Check sheet for the modelled part. Datum: model origin and axes. Units: mm. A direction names the side the tool comes from. Round coordinates to 2 decimals unless told otherwise and drop trailing zeros. Write each loop counter-clockwise with the first axis right and the second up, starting at its lowest first coordinate (ties: lowest second). Pieces come first, ordered by that corner, then holes.
Item 1: Go/stop test with flat-tipped pins: pin 1 Ø6 at (x, z) = (6.5, -2) entering from -Y; pin 2 Ø0.7 at (x, y) = (1.5, 1) entering from -Z; pin 3 Ø5 at (x, z) = (0, 0.5) entering from -Y; pin 4 Ø2.5 at (x, z) = (0, 0) entering from -Y (3 decimals). Record where each tip stops, or that it passes through.
Item 2: Tool access check on faces 5 (the flat face through (0, 5, -4.95)), 6 (the conical face through (0.025, 0.181, 1.144)). Record the directions out of +Z, -Z, +X, -X, +Y, -Y that give a thin tool (end or side, any length) a straight path to the whole face; none if there is none.
Item 3: Cross-section at A-A on x = 0. Enter the section's corners in (y, z) (3 decimals), plus the area to 3 significant figures.
Item 4: Cross-section at D-D on z = -10.5. Enter the section's corners in (x, y).
Item 5: Material ranges on line 1 (Z direction, x = -0.75, y = 6.5); line 2 (Y direction, x = -2.75, z = -6.25); line 3 (Y direction, x = 5.5, z = -1), recorded low to high.
Item 6: Release check for a two-part mould opening along Z. For faces 1 (the flat face through (-3.39, 5.24, 8.406)), 2 (the flat face through (0, 0, 2)), 3 (the cylindrical face through (0, 1.2, 2.5)), 4 (the flat face through (1.5, 1.2, 0.05)) record: +Z half, -Z half, draft (parallel to the pull), parting line (faces both ways), or undercut.
Item 7: Cross-section at B-B on x = -7.5. Enter the section's corners in (y, z).
Autodesk Inventor part; units mm, degrees
ref_plane "YZ Plane" through (0, 0, 0) normal (1, 0, 0) x (0, 1, 0)
ref_plane "XZ Plane" through (0, 0, 0) normal (0, 1, 0) x (-1, 0, 0)
ref_plane "XY Plane" through (0, 0, 0) normal (0, 0, 1) x (1, 0, 0)
sketch "Sketch1" plane through (0, 0, 0) normal (0, 0, 1) x (1, 0, 0)
  line L0 (0, 7) -> (0, 0) construction
  line L1 (0, 0) -> (1.025, 0) construction
  line L2 (1.025, 0) -> (1.025, 7)
  line L3 (1.025, 7) -> (0, 7) construction
  line L4 (1.025, 7) -> (12, 7)
  line L5 (3, 2.5) -> (2.5, 2.5)
  line L6 (2.5, 2.5) -> (2.5, 0)
  line L7 (2.5, 0) -> (1.025, 0)
  line L8 (12, 7) -> (12, 4.5)
  line L9 (12, 4.5) -> (3, 4.5)
  line L10 (3, 4.5) -> (3, 2.5)
  dimension "d0" = 2.5
  dimension "d1" = 1.025
  dimension "d3" = 0.5
  dimension "d4" = 2.5
  dimension "d9" = 2
  dimension "d10" = 12
  dimension "d11" = 2.5
revolve "Revolution1" add sketch "Sketch1" angle 360 about axis through (0, 7, 0) along (0, -1, 0)
sketch "Sketch2" plane through (0, 7, 0) normal (0, 1, 0) x (1, 0, 0)
  line L0 (0, 0) -> (0, 7.5) construction
  circle A0 centre (0, 7.5) radius 1.35
  line L1 (0, 0) -> (-7.1329, 2.3176) construction
  circle A1 centre (-7.1329, 2.3176) radius 1.35
  line L2 (0, 0) -> (-4.4084, -6.0676) construction
  circle A2 centre (-4.4084, -6.0676) radius 1.35
  line L3 (0, 0) -> (4.4084, -6.0676) construction
  circle A3 centre (4.4084, -6.0676) radius 1.35
  line L4 (0, 0) -> (7.1329, 2.3176) construction
  circle A4 centre (7.1329, 2.3176) radius 1.35
  dimension "d12" = 7.5
  dimension "d13" = 2.7
  dimension "d16" = 360
extrude "Extrusion1" cut sketch "Sketch2" against normal blind 10
sketch "Sketch3" plane through (0, 4.5, 0) normal (0, -1, 0) x (1, 0, 0)
  circle A0 centre (0, -7.5) radius 1.35 construction
  line L0 (-2.9445, -7.5) -> (-1.4722, -4.95)
  line L1 (-1.4722, -4.95) -> (1.4722, -4.95)
  line L2 (1.4722, -4.95) -> (2.9445, -7.5)
  line L3 (2.9445, -7.5) -> (1.4722, -10.05)
  line L4 (1.4722, -10.05) -> (-1.4722, -10.05)
  line L5 (-1.4722, -10.05) -> (-2.9445, -7.5)
  line L6 (6.223, -5.118) -> (4.2528, -2.9298)
  line L7 (4.2528, -2.9298) -> (5.1627, -0.1294)
  line L8 (5.1627, -0.1294) -> (8.0428, 0.4827)
  line L9 (8.0428, 0.4827) -> (10.0131, -1.7054)
  line L10 (10.0131, -1.7054) -> (9.1032, -4.5058)
  line L11 (9.1032, -4.5058) -> (6.223, -5.118)
  line L12 (6.7905, 4.3369) -> (4.1006, 3.1393)
  line L13 (4.1006, 3.1393) -> (1.7185, 4.87)
  line L14 (1.7185, 4.87) -> (2.0262, 7.7984)
  line L15 (2.0262, 7.7984) -> (4.7162, 8.996)
  line L16 (4.7162, 8.996) -> (7.0983, 7.2653)
  line L17 (7.0983, 7.2653) -> (6.7905, 4.3369)
  line L18 (-2.0262, 7.7984) -> (-1.7185, 4.87)
  line L19 (-1.7185, 4.87) -> (-4.1006, 3.1393)
  line L20 (-4.1006, 3.1393) -> (-6.7905, 4.3369)
  line L21 (-6.7905, 4.3369) -> (-7.0983, 7.2653)
  line L22 (-7.0983, 7.2653) -> (-4.7162, 8.996)
  line L23 (-4.7162, 8.996) -> (-2.0262, 7.7984)
  line L24 (-8.0428, 0.4827) -> (-5.1627, -0.1294)
  line L25 (-5.1627, -0.1294) -> (-4.2528, -2.9298)
  line L26 (-4.2528, -2.9298) -> (-6.223, -5.118)
  line L27 (-6.223, -5.118) -> (-9.1032, -4.5058)
  line L28 (-9.1032, -4.5058) -> (-10.0131, -1.7054)
  line L29 (-10.0131, -1.7054) -> (-8.0428, 0.4827)
  point P0 (0, 0)
  point P1 (0, -7.5)
  point P2 (7.1329, -2.3176)
  point P3 (7.1329, -2.3176)
  point P4 (4.4084, 6.0676)
  point P5 (4.4084, 6.0676)
  point P6 (-4.4084, 6.0676)
  point P7 (-4.4084, 6.0676)
  point P8 (-7.1329, -2.3176)
  point P9 (-7.1329, -2.3176)
  dimension "d20" = 5.1
  dimension "d23" = 360
extrude "Extrusion2" cut sketch "Sketch3" against normal blind 1.5
chamfer "Chamfer2" distance 0.3 angle 45 1 edges at (-1.025, 0, 0)
sketch "Sketch4" plane through (0, 0, 0) normal (0, -1, 0) x (1, 0, 0)
  line L0 (-3.3003, 0.05) -> (-3.3003, -4.3195)
  line L1 (-3.3003, -4.3195) -> (3.3085, -4.3195)
  line L2 (3.3085, -4.3195) -> (3.3085, 0.05)
  line L3 (3.3085, 0.05) -> (-3.3003, 0.05)
  point P0 (0, 0)
  point P1 (0, 0)
  dimension "d32" = 0.05
extrude "Extrusion3" cut sketch "Sketch4" against normal up to surface (2.5 mm away)
fillet "Fillet1" radius 0.5 2 edges at (2.4995, 1.25, 0.05) (-2.4995, 1.25, 0.05)
properties part number "Flywheel"
Response values:
1. pin 1: stops at y = 4.5
1. pin 2: stops at z = 0.05
1. pin 3: stops at y = 0
1. pin 4: stops at y = 0.075
2. face 5: -Y
2. face 6: -Z, -Y
3. outline: (0, 1.325) - (0.3, 1.025) - (7, 1.025) - (7, 12) - (4.5, 12) - (4.5, 3) - (2.5, 3) - (2.5, 2.5) - (0, 2.5) - close; (2.5, -3) - (4.5, -3) - (4.5, -4.95) - (6, -4.95) - (6, -6.15) - (7, -6.15) - (7, -1.025) - (2.5, -1.025) - close; (4.5, -12) - (7, -12) - (7, -8.85) - (6, -8.85) - (6, -10.05) - (4.5, -10.05) - close
3. area: 56.1 mm2
4. outline: (-5.81, 4.5) - (5.81, 4.5) - (5.81, 7) - (-5.81, 7) - close
5. line 1: z = -11.98 to -8.62, -6.38 to -0.7, 0.7 to 11.98
5. line 2: y = 4.5 to 7
5. line 3: y = 6 to 7
6. face 1: undercut
6. face 2: draft
6. face 3: +Z half
6. face 4: -Z half
7. outline: (4.5, -9.37) - (7, -9.37) - (7, -3.62) - (6, -3.62) - (6, -4.85) - (4.5, -4.85) - close; (4.5, 0.37) - (6, 0.37) - (6, -1.02) - (7, -1.02) - (7, 9.37) - (4.5, 9.37) - close
